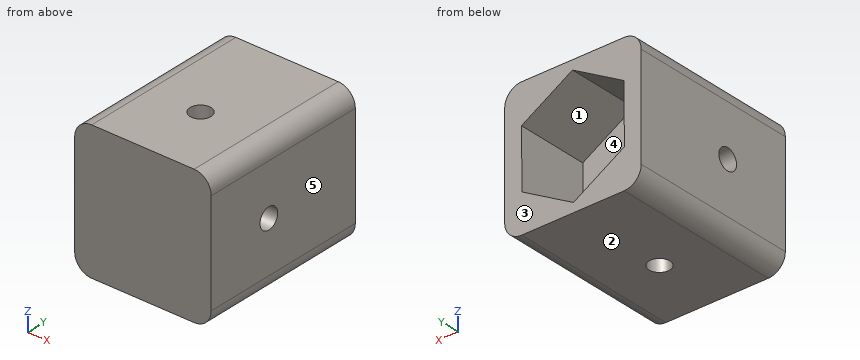
Autodesk Inventor part; units mm, degrees
ref_plane "YZ Plane" through (0, 0, 0) normal (1, 0, 0) x (0, 1, 0)
ref_plane "XZ Plane" through (0, 0, 0) normal (0, 1, 0) x (-1, 0, 0)
ref_plane "XY Plane" through (0, 0, 0) normal (0, 0, 1) x (1, 0, 0)
sketch "Sketch1" plane through (0, 0, 0) normal (0, 1, 0) x (-1, 0, 0)
  line L0 (0.0535, -6.928) -> (-5.9731, -3.5103)
  line L1 (-5.9731, -3.5103) -> (-6.0266, 3.4177)
  line L2 (-6.0266, 3.4177) -> (-0.0535, 6.928)
  line L3 (-0.0535, 6.928) -> (5.9731, 3.5103)
  line L4 (5.9731, 3.5103) -> (6.0266, -3.4177)
  line L5 (6.0266, -3.4177) -> (0.0535, -6.928)
  line L6 (6, 8) -> (-6, 8)
  line L7 (-8, 6) -> (-8, -6)
  line L8 (-6, -8) -> (6, -8)
  line L9 (8, -6) -> (8, 6)
  line L10 (8, 8) -> (-8, -8) construction
  line L11 (-8, 8) -> (8, -8) construction
  arc A0 (8, 6) -> (6, 8) centre (6, 6) ccw
  arc A1 (-6, 8) -> (-8, 6) centre (-6, 6) ccw
  arc A2 (-8, -6) -> (-6, -8) centre (-6, -6) ccw
  arc A3 (6, -8) -> (8, -6) centre (6, -6) ccw
  point P0 (0, 0)
  point P1 (0, 0)
  dimension "d0" = 12
  dimension "d1" = 16
  dimension "d2" = 16
  dimension "d7" = 2
extrude "Extrusion1" add sketch "Sketch1" along normal blind 8.5
extrude "Extrusion2" add sketch "Sketch1" against normal blind 11.5 contours L0 L1 L2 L3 L4 L5 | A0 L9 A3 L8 A2 L7 A1 L6
sketch "Sketch2" plane through (8, 8.5, 6) normal (1, 0, 0) x (0, 0, -1)
  line L0 (12, -20) -> (12, 0)
  line L1 (0, 0) -> (12, 0)
  line L2 (0, -20) -> (0, 0)
  line L3 (12, -20) -> (0, -20)
  point P0 (6, -8.5)
  point P1 (6, -12)
  point P2 (6, -20)
  dimension "d8" = 12
hole "Hole1" at (8, -3.5, 0) direction (-1, 0, 0) diameter 2.45 depth 3 tip angle 118
pattern_circular "Circular Pattern1" count 4 over 360 about axis through (0, -10, 0) along (0, 1, 0) of "Hole1"
properties part number "couplingload"
Verification items for the finished model (mm, model axes). Face numbers are marked on the shaded views. A direction names the side the tool comes from. Give positions to 0.01 mm unless a question says otherwise; leave off trailing zeros. Order: outer loops, then holes, each group sorted by start corner. A loop starts at its lowest first (then second) coordinate and runs counter-clockwise, first axis right, second up. Notation, with made-up numbers: M 78.5,21 L 104.5,21 A22 cw 104.5,27 Z; hole C 50.25,46.5 d7. An arc over 180 degrees is marked long. Answer as a JSON object with one key per item and string values. Group by question number.
1) Access from +Z, -Z, +X, -X, +Y, -Y to the whole of each face (thin tool, end or side, straight path). Record for the marked faces 4 and 5.
2) Scan lines: line 1 along Y through (x, z) = (5.85, 0) (3 decimals); line 2 along Y through (x, z) = (0, 7.4) (3 decimals); line 3 along X through (y, z) = (1, -0.5). Record each from-to range of solid material in increasing order. Write a range as [from, to].
3) Cross-section at C-C (x = 2.5). Enter the section's corners in (y, z), then the cut area to 3 significant figures.
4) Mould release check, pull along Z, two halves, no side actions. Record for the marked faces 1, 2 and 3: released by +Z, released by -Z, zero draft, split by the parting line, or undercut.
5) Cross-section at B-B (z = 2.5). Enter the section's corners in (x, y).
6) Cross-section at A-A (y = 4). Enter the section's corners in (x, z).
7) Depth check by flat-ended pin: pin 1 Ø2 at (y, z) = (-3.5, 0) entering from +X; pin 2 Ø1.5 at (x, y) = (0, -3.5) entering from +Z; pin 3 Ø1 at (x, z) = (-2, 3) entering from +Y. Enter the tip coordinate at first touch or a pass-through.
Result sheet:
{
 "1": {"face 4": "+Y", "face 5": "+Z, -Z, +X, +Y, -Y"},
 "2": {"line 1": "y = [-11.5, -4.725], [-2.275, 0]", "line 2": "y = [-11.5, -4.725], [-2.275, 8.5]", "line 3": "x = [-8, -6], [6, 8]"},
 "3": {"outline": "M -11.5,-8 L 8.5,-8 L 8.5,-5.48 L 0,-5.48 L 0,5.49 L 8.5,5.49 L 8.5,8 L -11.5,8 Z", "area": "227 mm2"},
 "4": {"face 1": "undercut", "face 2": "released by -Z", "face 3": "zero draft"},
 "5": {"outline": "M -8,-11.5 L 8,-11.5 L 8,8.5 L 6.02,8.5 L 6.02,0 L -5.98,0 L -5.98,8.5 L -8,8.5 Z"},
 "6": {"outline": "M -8,-6 A2 ccw -6,-8 L 6,-8 A2 ccw 8,-6 L 8,6 A2 ccw 6,8 L -6,8 A2 ccw -8,6 Z; hole M -6.03,-3.42 L -0.05,-6.93 L 5.97,-3.51 L 6.03,3.42 L 0.05,6.93 L -5.97,3.51 Z"},
 "7": {"pin 1": "stops at x = 4.86", "pin 2": "stops at z = 4.71", "pin 3": "stops at y = 0"}
}
